For this review, take the finished solid that the model builds, in its own axes (mm). A direction names the side the tool comes from. Coordinates: 2 decimals unless noted, no trailing zeros. Loops run counter-clockwise (first coordinate to the right, second up) from the corner with the lowest first, then second, coordinate; pieces in that order, holes last. Notation, with made-up numbers: (61, -21.75) -> (93, -21.75) arc R26 cw to (93, -0.75) -> close; hole circle Ø11 at (66, -13.5). An arc over 180 degrees is marked (long way). One line per item, written item: value.
from build123d import *

# Parameters (mm, degrees)
PAD001_DEPTH    = 2.8
POCKET005_DEPTH = 2.801
SKETCH021_W     = 12.7
SKETCH021_H     = 1.6
POCKET010_DEPTH = 2.801
SKETCH022_R     = 0.25
POCKET011_DEPTH = 2.801


with BuildPart() as part:
    # Sketch001 (on Face18 of ShapeBinder) → Pad001 (new body)
    with BuildSketch(Plane.YZ.offset(35)):
        Polygon((-22.588718, 60.327675), (17.411282, 60.327675), (17.411282, -34.672325), (-57.588718, -34.672325), (-57.588718, 0.327675), (-23.239438, 0.327675), (-7.588718, 43.327675), (-22.588718, 43.327675), align=None)
        with BuildLine():
            ThreePointArc((-12.161797, -2.94822), (-14.851323, 2.819487), (-20.61903, 0.129961))
            Line((-20.61903, 0.129961), (-23.697212, -8.327272))
            ThreePointArc((-23.697212, -8.327272), (-21.007685, -14.09498), (-15.239978, -11.405454))
            Line((-15.239978, -11.405454), (-12.161797, -2.94822))
        make_face(mode=Mode.SUBTRACT)
        with BuildLine():
            ThreePointArc((-3.468033, -5.876244), (-5.261051, -2.031105), (-9.106189, -3.824123))
            Line((-9.106189, -3.824123), (-12.18437, -12.281356))
            ThreePointArc((-12.18437, -12.281356), (-10.391353, -16.126495), (-6.546214, -14.333477))
            Line((-6.546214, -14.333477), (-3.468033, -5.876244))
        make_face(mode=Mode.SUBTRACT)
        Polygon((10.819102, 21.538585), (13.450241, 20.580929), (7.057884, 3.018073), (4.426745, 3.97573), align=None, mode=Mode.SUBTRACT)
        Polygon((1.006544, -5.421196), (3.637683, -6.378853), (-2.754673, -23.941708), (-5.385813, -22.984051), align=None, mode=Mode.SUBTRACT)
    extrude(amount=PAD001_DEPTH)

    # Sketch013 (on Face26 of Pad001) → Pocket005 (cut, through all)
    with BuildSketch(Plane.YZ.offset(37.8)):
        with BuildLine():
            ThreePointArc((1.252746, -5.377784), (0.900889, -5.194619), (0.815033, -5.581893))
            ThreePointArc((0.858445, -5.828095), (0.869723, -5.699178), (0.815033, -5.581893))
            Line((0.858445, -5.828095), (1.413442, -5.569295))
            ThreePointArc((1.252746, -5.377784), (1.307436, -5.495069), (1.413442, -5.569295))
        make_face()
        with BuildLine():
            ThreePointArc((3.681095, -6.625055), (3.86426, -6.273198), (3.476986, -6.187342))
            ThreePointArc((3.230784, -6.230754), (3.359701, -6.242032), (3.476986, -6.187342))
            Line((3.489584, -6.785752), (3.230784, -6.230754))
            ThreePointArc((3.681095, -6.625055), (3.56381, -6.679746), (3.489584, -6.785752))
        make_face()
        with BuildLine():
            ThreePointArc((-5.429225, -22.737849), (-5.61239, -23.089706), (-5.225116, -23.175563))
            ThreePointArc((-4.978914, -23.13215), (-5.107831, -23.120872), (-5.225116, -23.175563))
            Line((-5.237714, -22.577153), (-4.978914, -23.13215))
            ThreePointArc((-5.429225, -22.737849), (-5.31194, -22.683159), (-5.237714, -22.577153))
        make_face()
        with BuildLine():
            ThreePointArc((-3.000875, -23.98512), (-2.649019, -24.168285), (-2.563162, -23.781011))
            ThreePointArc((-2.606574, -23.534809), (-2.617853, -23.663726), (-2.563162, -23.781011))
            Line((-2.606574, -23.534809), (-3.161572, -23.793609))
            ThreePointArc((-3.000875, -23.98512), (-3.055566, -23.867835), (-3.161572, -23.793609))
        make_face()
        with BuildLine():
            ThreePointArc((11.065304, 21.581997), (10.713447, 21.765162), (10.62759, 21.377888))
            ThreePointArc((10.671003, 21.131686), (10.682281, 21.260603), (10.62759, 21.377888))
            Line((10.671003, 21.131686), (11.226, 21.390486))
            ThreePointArc((11.065304, 21.581997), (11.119994, 21.464712), (11.226, 21.390486))
        make_face()
        with BuildLine():
            ThreePointArc((13.493653, 20.334727), (13.676818, 20.686583), (13.289544, 20.77244))
            ThreePointArc((13.043342, 20.729028), (13.172259, 20.717749), (13.289544, 20.77244))
            Line((13.302142, 20.17403), (13.043342, 20.729028))
            ThreePointArc((13.493653, 20.334727), (13.376368, 20.280036), (13.302142, 20.17403))
        make_face()
        with BuildLine():
            ThreePointArc((4.383333, 4.221932), (4.200168, 3.870075), (4.587442, 3.784219))
            ThreePointArc((4.833644, 3.827631), (4.704727, 3.83891), (4.587442, 3.784219))
            Line((4.574844, 4.382629), (4.833644, 3.827631))
            ThreePointArc((4.383333, 4.221932), (4.500618, 4.276623), (4.574844, 4.382629))
        make_face()
        with BuildLine():
            ThreePointArc((6.811682, 2.974661), (7.163539, 2.791497), (7.249396, 3.17877))
            ThreePointArc((7.205983, 3.424972), (7.194705, 3.296055), (7.249396, 3.17877))
            Line((7.205983, 3.424972), (6.650986, 3.166173))
            ThreePointArc((6.811682, 2.974661), (6.756992, 3.091946), (6.650986, 3.166173))
        make_face()
    extrude(amount=-POCKET005_DEPTH, mode=Mode.SUBTRACT)

    # Sketch021 (on Face5 of Pocket005) → Pocket010 (cut, through all)
    with BuildSketch(Plane.YZ.offset(37.8)):
        with Locations((-44.116, -5.2)):
            Rectangle(SKETCH021_W, SKETCH021_H)
    extrude(amount=-POCKET010_DEPTH, mode=Mode.SUBTRACT)

    # Sketch022 (on Face5 of Pocket010) → Pocket011 (cut, through all)
    with BuildSketch(Plane.YZ.offset(37.8)):
        with Locations((-50.466, -4.4)):
            Circle(SKETCH022_R)
        with Locations((-37.766, -4.4)):
            Circle(SKETCH022_R)
        with Locations((-37.766, -6)):
            Circle(SKETCH022_R)
        with Locations((-50.466, -6)):
            Circle(SKETCH022_R)
    extrude(amount=-POCKET011_DEPTH, mode=Mode.SUBTRACT)


solid = part.part
1. For faces 4 (the flat face through (36.38, -15.524, 21.527)), 5 (the flat face through (36, -41, 0.328)), 6 (the flat face through (36, -44, -4.4)), 7 (the flat face through (35, -11, 3)), list the 3-axis set-ups (+Z, -Z, +X, -X, +Y, -Y) from which the entire face can be reached by the end or side of a thin tool; tool diameter is ignored.
Return value:
face 4: +X, -X, -Y
face 5: +Z, +X, -X, -Y
face 6: +X, -X
face 7: +Z, -Z, -X, +Y, -Y
2. Take a section at A-A, the plane z = 13. Give the boundary of the cut face in (x, y).
Return value:
outline: (35, -18.63) -> (37.8, -18.63) -> (37.8, 7.71) -> (35, 7.71) -> close; (35, 10.69) -> (37.8, 10.69) -> (37.8, 17.41) -> (35, 17.41) -> close
3. Take a section at B-B, the plane x = 36.95. Give the number of separate pieces and of enclosed holes in the cut face, and give its area (3 significant figures).
Return value:
separate pieces: 1
enclosed holes: 5
area: 4,360 mm2
4. Take a section at C-C, the plane z = -21.5. Give the boundary of the cut face in (x, y).
Return value:
outline: (35, -57.59) -> (37.8, -57.59) -> (37.8, -4.85) -> (35, -4.85) -> close; (35, -1.87) -> (37.8, -1.87) -> (37.8, 17.41) -> (35, 17.41) -> close
5. Take a section at D-D, the plane z = 53. Give the boundary of the cut face in (x, y), and give its area (3 significant figures).
Return value:
outline: (35, -22.59) -> (37.8, -22.59) -> (37.8, 17.41) -> (35, 17.41) -> close
area: 112 mm2
6. Insertion check: pin 1 Ø1.4 at (x, z) = (36, 52.5) entering from -Y; pin 2 Ø0.8 at (x, y) = (36, -41.5) entering from +Z. Each pin has a flat end and moves straight along its axis. Give the tip position at first contact, or say it passes through.
Return value:
pin 1: stops at y = -22.59
pin 2: stops at z = 0.33
7. The part is to be moulded in two halves that separate along Z. For faces 1 (the flat face through (36, -22.589, 52)), 2 (the flat face through (36, -3, 60.328)), 3 (the flat face through (36.38, -2.232, -14.32)), say which applies: pulls with the +Z half, pulls with the -Z half, needs draft (parallel to the pull), parting line crosses it, or undercut.
Return value:
face 1: needs draft
face 2: pulls with the +Z half
face 3: undercut
8. To check wall thickness, follow probe 1 along Z at (x, y) = (36.2, -49); probe 2 along Y at (x, z) = (35.45, -3); probe 3 along Y at (x, z) = (37.05, -6.5). State the ranges of each line that lie inside material, in increasing order. Write a range as from..to.
Return value:
probe 1: z = -34.67..-6, -4.4..0.33
probe 2: y = -57.59..-21.76, -12.18..-8.65, -3.93..17.41
probe 3: y = -57.59..-23.03, -13.45..-10.08, -3.7..0.61, 3.86..17.41
